Read the model definition and answer for the solid it produces. Units are mm, in the model's axes. A direction names the side the tool comes from. Round coordinates to 2 decimals unless told otherwise and drop trailing zeros. Order: outer loops, then holes, each group sorted by start corner. A loop starts at its lowest first (then second) coordinate and runs counter-clockwise, first axis right, second up. Notation, with made-up numbers: (77.25, 16.5) - (87.25, 16.5) arc R14 cw to (87.25, 22.5) - close; hole circle Ø2 at (-23, -1). An arc over 180 degrees is marked (long way). Answer as a JSON object with one key per item and string values. Group by question number.
Q1. Consider line 1 (Z direction, x = -7, y = 0.5); line 2 (Z direction, x = -11.75, y = 28.5); line 3 (Z direction, x = -5.75, y = 44.5). Determine where each line is inside the solid, lowest interval first.
Q2. The mould has two halves that part along Y. Classify faces 1 (the cylindrical face through (-1, 7.7, -14)), 2 (the flat face through (-7, 2, -8)), 3 (the cylindrical face through (-17.04, 0.99, -8.84)): pulls with the +Y half, pulls with the -Y half, needs draft (parallel to the pull), parting line crosses it, or undercut.
Q3. A cutting plane is placed at C-C on y = 14.5. Determine the outline of the cut face in (x, z).
Q4. A cutting plane is placed at B-B on z = -18.5. Determine the outline of the cut face in (x, y), and give its area (3 significant figures).
Q5. A cutting plane is placed at A-A on x = 2.5. Determine the outline of the cut face in (y, z), and give its area (3 significant figures).
Q6. Given pin 1 Ø1.6 at (y, z) = (1, -18.5) entering from +X; pin 2 Ø4 at (x, y) = (-6, 24.5) entering from -Z; pin 3 Ø2.5 at (x, z) = (3, -7) entering from +Y; pin 4 Ø1.6 at (x, z) = (2.5, -8) entering from +Y, each flat-ended and moving along its own axis, determine where each tip first touches the part or whether it passes through.
Q7. A tool of negligible diameter and unlimited length cuts with its end or side. For faces 4 (the flat face through (-12.5, 50, -8)), 5 (the flat face through (-5.85, 2, 2.54)), 6 (the flat face through (-4.5, 1, 3)), 7 (the flat face through (-17, 1, -5.5)), from which of +Z, -Z, +X, -X, +Y, -Y can it reach the whole face along a straight path? Write none if from no direction.
Q8. A cutting plane is placed at D-D on x = -7. Determine the outline of the cut face in (y, z).
Autodesk Inventor part; units mm, degrees
ref_plane "YZ Plane" through (0, 0, 0) normal (1, 0, 0) x (0, 1, 0)
ref_plane "XZ Plane" through (0, 0, 0) normal (0, 1, 0) x (-1, 0, 0)
ref_plane "XY Plane" through (0, 0, 0) normal (0, 0, 1) x (1, 0, 0)
sketch "Boceto1" plane through (0, 0, 0) normal (0, 1, 0) x (-1, 0, 0)
  line L0 (0, 0) -> (14, 0)
  line L1 (14, 0) -> (14, -16)
  line L2 (14, -16) -> (0, -16)
  line L3 (0, -16) -> (0, 0)
  line L4 (12, -2) -> (2, -2)
  line L5 (2, -2) -> (2, -14)
  line L6 (2, -14) -> (12, -14)
  line L7 (12, -14) -> (12, -2)
  line L8 (12, -2) -> (2, -14) construction
  line L9 (2, -2) -> (12, -14) construction
  line L10 (14, -8) -> (14, -10.5)
  line L11 (14, -10.5) -> (19, -10.5)
  line L12 (19, -10.5) -> (19, -5.5)
  line L13 (19, -5.5) -> (14, -5.5)
  circle A0 centre (16.5, -8) radius 1
  line L14 (7, -16) -> (4.5, -16)
  line L15 (4.5, -16) -> (4.5, -21)
  line L16 (4.5, -21) -> (9.5, -21)
  line L17 (9.5, -21) -> (9.5, -16)
  circle A1 centre (7, -18.5) radius 1
  line L18 (7, 0) -> (9.5, 0)
  line L19 (9.5, 0) -> (9.5, 5)
  line L20 (9.5, 5) -> (4.5, 5)
  line L21 (4.5, 5) -> (4.5, 0)
  circle A2 centre (7, 2.5) radius 1
  line L22 (0, -8) -> (0, -10.5)
  line L23 (0, -10.5) -> (-5, -10.5)
  line L24 (-5, -10.5) -> (-5, -5.5)
  line L25 (-5, -5.5) -> (0, -5.5)
  circle A3 centre (-2.5, -8) radius 1
  point P0 (7, -8)
  dimension "d0" = 14
  dimension "d1" = 16
  dimension "d2" = 10
  dimension "d3" = 12
  dimension "d4" = 2.5
  dimension "d5" = 5
  dimension "d6" = 5
  dimension "d7" = 2
  dimension "d8" = 2.5
  dimension "d9" = 5
  dimension "d10" = 5
  dimension "d11" = 2
  dimension "d12" = 2.5
  dimension "d13" = 5
  dimension "d14" = 5
  dimension "d15" = 2
  dimension "d16" = 2.5
  dimension "d17" = 5
  dimension "d18" = 5
  dimension "d19" = 2
extrude "Extrusión1" add sketch "Boceto1" along normal blind 2
sketch "Boceto2" plane through (0, 2, 0) normal (0, 1, 0) x (1, 0, 0)
  line L0 (-9.5, 16) -> (-14, 16)
  line L1 (-14, 16) -> (0, 16)
  line L2 (0, 16) -> (0, 0)
  line L3 (-14, 0) -> (-9.5, 0)
  line L4 (0, 0) -> (-14, 0)
  line L5 (-14, 16) -> (-14, 10.5)
  line L6 (-14, 0) -> (-14, 16)
  line L7 (-2, 14) -> (-12, 14)
  line L8 (-12, 14) -> (-12, 1.9304)
  line L9 (-12, 1.9304) -> (-2, 1.9304)
  line L10 (-2, 14) -> (-2, 2)
  line L11 (-2, 1.9304) -> (-2, 14)
  line L12 (-2, 14) -> (-12, 14)
extrude "Extrusión2" add sketch "Boceto2" along normal blind 62
sketch "Boceto3" plane through (0, 0, -10.5) normal (1, 0, 0) x (0, 0, -1)
  line L0 (-5, 7.8078) -> (0, 7.8078) construction
  line L1 (-5, 4.3078) -> (0, 4.3078)
  line L2 (0, 11.3078) -> (-5, 11.3078)
  arc A0 (-5, 11.3078) -> (-5, 4.3078) centre (-5, 7.8078) ccw
  arc A1 (0, 4.3078) -> (0, 11.3078) centre (0, 7.8078) ccw
  line L3 (3.5, 0) -> (3.5, 64)
  point P0 (-10.5, 0)
  point P1 (-2.5, 7.8078)
extrude "Extrusión3" cut sketch "Boceto3" against normal blind 2
extrude "Extrusión4" add sketch "Boceto1" along normal blind 2 contours L7 L6 L5 L4
sketch "Boceto4" plane through (0, 64, 0) normal (0, 1, 0) x (1, 0, 0)
  line L0 (-12, 14) -> (-2, 14)
  line L1 (-12, 14) -> (-2, 14)
  line L2 (-2, 2) -> (-2, 5.5)
  line L3 (-2, 14) -> (-2, 2)
  line L4 (-2, 1.9304) -> (-12, 1.9304)
  line L5 (-2, 2) -> (-12, 1.9304)
  line L6 (-12, 1.9304) -> (-12, 14)
  line L7 (-12.5, 14.4652) -> (-1.5, 14.4652)
  line L8 (-1.5, 14.4652) -> (-1.5, 1.4652)
  line L9 (-1.5, 1.4652) -> (-12.5, 1.4652)
  line L10 (-12.5, 1.4652) -> (-12.5, 14.4652)
  line L11 (-12.5, 14.4652) -> (-1.5, 1.4652) construction
  line L12 (-1.5, 14.4652) -> (-12.5, 1.4652) construction
  point P0 (0, 0)
  point P1 (-7, 7.9652)
  dimension "d28" = 11
  dimension "d29" = 13
extrude "Extrusión5" cut sketch "Boceto4" against normal blind 28
properties part number "SoporteMotorx1"
Result set:
{
 "1": {"line 1": "z = -21 to -19.5, -17.5 to 1.5, 3.5 to 5", "line 2": "z = -16 to -14, -1.93 to 0", "line 3": "z = -16 to -14.47, -1.47 to 0"},
 "2": {"face 1": "undercut", "face 2": "pulls with the +Y half", "face 3": "needs draft"},
 "3": {"outline": "(-14, -16) - (0, -16) - (0, 0) - (-14, 0) - close; hole (-12, -14) - (-2, -14) - (-2, -1.93) - (-12, -1.93) - close"},
 "4": {"outline": "(-9.5, 0) - (-8, 0) - (-8, 2) - (-9.5, 2) - close; (-6, 0) - (-4.5, 0) - (-4.5, 2) - (-6, 2) - close", "area": "6.00 mm²"},
 "5": {"outline": "(0, -10.5) - (2, -10.5) - (2, -9) - (0, -9) - close; (0, -7) - (2, -7) - (2, -5.5) - (0, -5.5) - close", "area": "6.00 mm²"},
 "6": {"pin 1": "stops at x = -4.5", "pin 2": "stops at z = -16", "pin 3": "stops at y = 2", "pin 4": "passes through"},
 "7": {"face 4": "+Y", "face 5": "+Z, +X, -X, +Y", "face 6": "+Z, +X, +Y, -Y", "face 7": "+Z, -X, +Y, -Y"},
 "8": {"outline": "(0, -21) - (2, -21) - (2, -19.5) - (0, -19.5) - close; (0, -17.5) - (2, -17.5) - (2, -16) - (64, -16) - (64, -14.47) - (36, -14.47) - (36, -14) - (2, -14) - (2, -1.93) - (36, -1.93) - (36, -1.47) - (64, -1.47) - (64, 0) - (2, 0) - (2, 1.5) - (0, 1.5) - close; (0, 3.5) - (2, 3.5) - (2, 5) - (0, 5) - close"}
}
